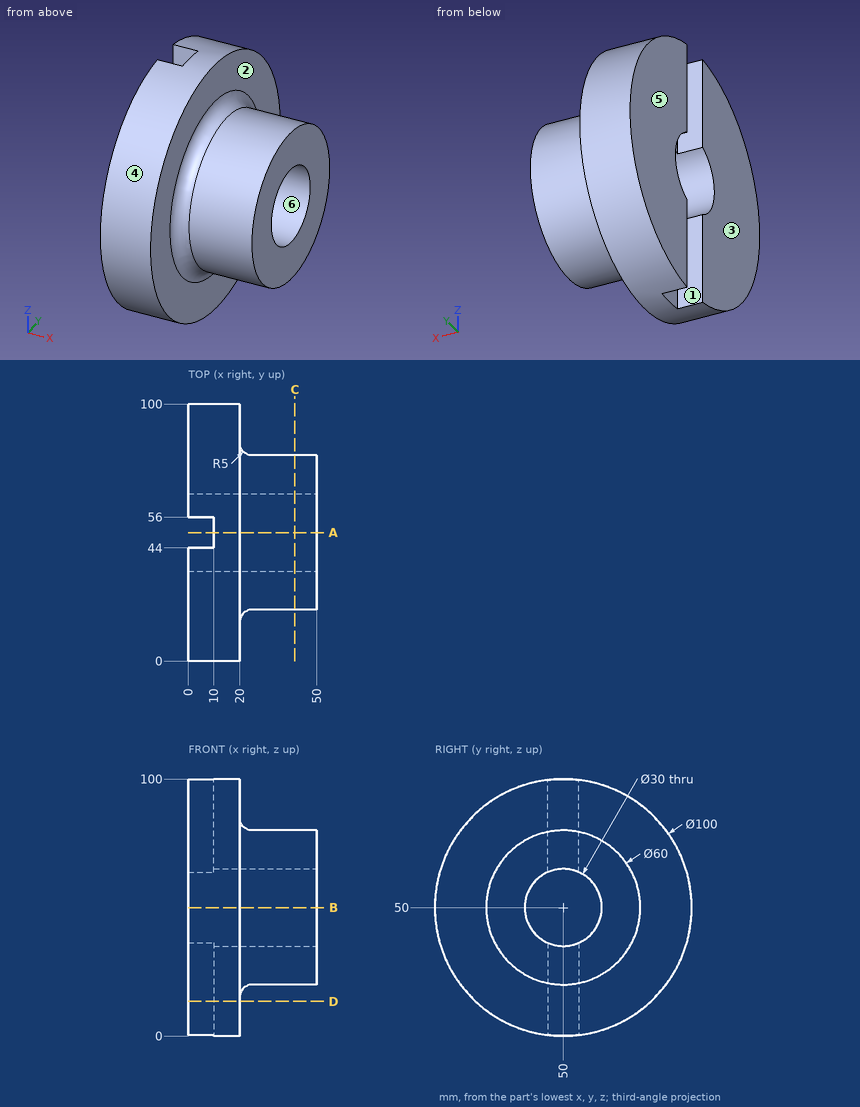
Input: dimensioned drawing with shaded views. Units: mm. Origin: part minimum x, y, z. A direction names the side the tool comes from. Round coordinates to 2 decimals unless told otherwise and drop trailing zeros. Loops run counter-clockwise (first coordinate to the right, second up) from the corner with the lowest first, then second, coordinate; pieces in that order, holes last. Notation, with made-up numbers: M 33,-32 L 57,-32 A23 cw 57,-24 Z; hole C 21.5,-16 d10. An arc over 180 degrees is marked long. Answer in a Markdown table with one row per item. Add a question column.
1. Section D-D (z = 13.5). Output: boundary loops of the cut face in (x, y).
2. Section A-A (y = 50). Output: boundary loops of the cut face in (x, z), and give its area (3 significant figures).
3. Ray query, probe 1 along Z at (x, y) = (37, 50); probe 2 along Z at (x, y) = (17, 50); probe 3 along X at (y, z) = (69.5, 7.5). Return the intervals inside material, ascending.
4. Set-up query: the marked faces 1, 2 and 3. Return all of +Z, -Z, +X, -X, +Y, -Y with unobstructed straight access to the full face (end or side cutting, diameter ignored); none if empty.
5. Section C-C (x = 41.5). Output: boundary loops of the cut face in (y, z), and give its area (3 significant figures).
6. Mould query, pull axis Y, two halves, no side actions, for the marked faces 4, 5 and 6. Classes: released by +Y, released by -Y, zero draft, split by the parting line, or undercut.
7. Contact query for flat-ended pins moving along their axis: pin 1 (4 mm diameter, centred on x = 19.5, y = 76, fed in from -Z); pin 2 (8 mm diameter, centred on x = 8, y = 76.5, fed in from -Z); pin 3 (8 mm diameter, centred on x = 19.5, y = 46.5, fed in from +Z). Output: stop coordinate, or through.
8. Section B-B (z = 50). Output: boundary loops of the cut face in (x, y).
Values follow:
| question | item | result |
|---|---|---|
| 1 | outline | M 0,15.83 L 20,15.83 L 20,84.17 L 0,84.17 L 0,56 L 10,56 L 10,44 L 0,44 Z |
| 2 | outline | M 10,0 L 20,0 L 20,15 A5 cw 25,20 L 50,20 L 50,35 L 10,35 Z; M 10,65 L 50,65 L 50,80 L 25,80 A5 cw 20,85 L 20,100 L 10,100 Z |
| 2 | area | 1,610 mm^2 |
| 3 | probe 1 | 20 to 35, 65 to 80 |
| 3 | probe 2 | 0 to 35, 65 to 100 |
| 3 | probe 3 | 0 to 20 |
| 4 | face 1 | +Z, -Z, -X |
| 4 | face 2 | +X |
| 4 | face 3 | +Z, -Z, -X, +Y, -Y |
| 5 | outline | C 50,50 d60; hole C 50,50 d30 |
| 5 | area | 2,120 mm^2 |
| 6 | face 4 | split by the parting line |
| 6 | face 5 | zero draft |
| 6 | face 6 | undercut |
| 7 | pin 1 | z = 6.14 |
| 7 | pin 2 | z = 5.35 |
| 7 | pin 3 | z = 100 |
| 8 | outline | M 0,0 L 20,0 L 20,15 A5 cw 25,20 L 50,20 L 50,35 L 0,35 Z; M 0,65 L 50,65 L 50,80 L 25,80 A5 cw 20,85 L 20,100 L 0,100 Z |
